Verification items for the finished model (mm, model axes). A direction names the side the tool comes from. Give positions to 0.01 mm unless a question says otherwise; leave off trailing zeros. Write each loop counter-clockwise with the first axis right and the second up, starting at its lowest first coordinate (ties: lowest second). Pieces come first, ordered by that corner, then holes. Notation, with made-up numbers: (3, 2.5) - (60, 2.5) arc R23 cw to (60, 18.5) - close; hole circle Ø3 at (-19, 54.5). An arc over 180 degrees is marked (long way). Put each result on its own line as item: value.
from build123d import *

# Parameters (mm, degrees)
EXTRUDE1_DEPTH     = 25.4
SKETCH2_R          = 9.36
SKETCH2_R_2        = 8
SKETCH2_R_3        = 1.55
CUT_EXTRUDE1_DEPTH = 77.2
SKETCH3_R          = 11
CUT_EXTRUDE2_DEPTH = 2
SKETCH4_R          = 1.55
SKETCH4_W          = 3.14
SKETCH4_H          = 15.875
SKETCH4_W_2        = 3.2
CUT_EXTRUDE3_DEPTH = 77.2


with BuildPart() as part:
    # Sketch1 → Extrude1 (new body)
    with BuildSketch(Plane.XY):
        Polygon((0, 0), (50.8, 0), (50.8, 3.14), (3.14, 3.14), (3.14, 50.8), (0, 50.8), align=None)
    extrude(amount=EXTRUDE1_DEPTH)

    # Sketch2 → Cut-Extrude1 (cut, through all)
    with BuildSketch(Plane.ZY):
        with Locations((12.7, 11.1125)):
            Circle(SKETCH2_R)
        with Locations((12.7, 38.4725)):
            Circle(SKETCH2_R_2)
        with Locations((4.7625, 23.8125)):
            Circle(SKETCH2_R_3)
        with Locations((20.6375, 23.8125)):
            Circle(SKETCH2_R_3)
    extrude(amount=-CUT_EXTRUDE1_DEPTH, mode=Mode.SUBTRACT)

    # Sketch3 → Cut-Extrude2 (cut)
    with BuildSketch(Plane(origin=(3.14, 0, 0), x_dir=(0, 0, -1), z_dir=(1, 0, 0))):
        with Locations((-12.7, 38.4725)):
            Circle(SKETCH3_R)
    extrude(amount=-CUT_EXTRUDE2_DEPTH, mode=Mode.SUBTRACT)

    # Sketch4 → Cut-Extrude3 (cut, through all)
    with BuildSketch(Plane.XZ):
        with Locations(Location((12.7, 12.7, 0), (0, 0, 270))):
            Circle(SKETCH4_R)
        with Locations(Location((42.86, 12.7, 0), (0, 0, 270))):
            Circle(SKETCH4_R)
        with Locations((7.71, 12.7)):
            Rectangle(SKETCH4_W, SKETCH4_H)
        with Locations((48.04, 12.7)):
            Rectangle(SKETCH4_W_2, SKETCH4_H)
    extrude(amount=-CUT_EXTRUDE3_DEPTH, mode=Mode.SUBTRACT)


solid = part.part
Q1. Go/stop test with flat-tipped pins: pin 1 Ø2.5 at (x, z) = (33.5, 20.5) entering from +Y; pin 2 Ø5 at (y, z) = (23.81, 20.64) entering from +X. Record where each tip stops, or that it passes through.
Answers follow:
pin 1: stops at y = 3.14
pin 2: stops at x = 3.14
Q2. Release check for a two-part mould opening along Y. For faces 1 (the face through (2.3, 2.8, 17)), 2 (the face through (1.55, 25.35, 4.56)), 3 (the face through (50.8, 1.5, 12.5)), 4 (the face through (2, 50.8, 13)) record: released by +Y, released by -Y, zero draft, split by the parting line, or undercut.
Answers follow:
face 1: undercut
face 2: undercut
face 3: zero draft
face 4: released by +Y
Q3. Section check A-A, the plane z = 12.7. Give the number of separate pieces and of enclosed holes in the cut face, plus the area to 3 significant figures.
Answers follow:
separate pieces: 7
enclosed holes: 0
area: 100 mm2
Q4. Section check D-D, the plane x = 42.86. Record the cut outline in (y, z).
Answers follow:
outline: (0, 0) - (3.14, 0) - (3.14, 7.8) arc R9.36 cw to (1.88, 11.15) - (0, 11.15) - close; (0, 14.25) - (1.88, 14.25) arc R9.36 cw to (3.14, 17.6) - (3.14, 25.4) - (0, 25.4) - close
Q5. Section check B-B, the plane x = 7. Record the cut outline in (y, z).
Answers follow:
outline: (0, 0) - (3.14, 0) - (3.14, 4.76) - (0, 4.76) - close; (0, 20.64) - (3.14, 20.64) - (3.14, 25.4) - (0, 25.4) - close
Q6. Section check C-C, the plane y = 44. Record the cut outline in (x, z), plus the area to 3 significant figures.
Answers follow:
outline: (0, 0) - (3.14, 0) - (3.14, 3.19) - (1.14, 3.19) - (1.14, 6.92) - (0, 6.92) - close; (0, 18.48) - (1.14, 18.48) - (1.14, 22.21) - (3.14, 22.21) - (3.14, 25.4) - (0, 25.4) - close
area: 28.5 mm2
Q7. Scan lines: line 1 along Y through (x, z) = (0.7, 12.7); line 2 along X through (y, z) = (1.1, 12.7); line 3 along Y through (x, z) = (2.5, 12.7). Record each from-to range of solid material in increasing order.
Answers follow:
line 1: y = 0 to 1.75, 20.47 to 30.47, 46.47 to 50.8
line 2: x = 0 to 6.14, 9.28 to 11.15, 14.25 to 41.31, 44.41 to 46.44, 49.64 to 50.8
line 3: y = 0 to 1.75, 20.47 to 27.47, 49.47 to 50.8
Q8. Set-up check for faces 5 (the face through (46.44, 1, 13)), 6 (the face through (50.212, 1.753, 12.628)), 7 (the face through (3.14, 27, 13)): record each of +Z, -Z, +X, -X, +Y, -Y from which the full face is reachable in a straight line by a thin tool's end or side.
Answers follow:
face 5: +Y, -Y
face 6: +X, -X, +Y
face 7: +Z, -Z, +X, +Y
